```python
from build123d import *

# Parameters (mm, degrees)
SKETCH1_W           = 7
SKETCH1_H           = 2
SKETCH1_R           = 1
SKETCH1_W_2         = 23.5
SKETCH1_H_2         = 13
BOSS_EXTRUDE1_DEPTH = 2


with BuildPart() as part:
    # Sketch1 → Boss-Extrude1 (new body)
    with BuildSketch(Plane(origin=(0, 0, 0), x_dir=(1, 0, 0), z_dir=(0, 1, 0))):
        Polygon((66.949898611, 13.823848353), (-23.050101389, 13.823848353), (-23.050101389, 8.823848353), (-25.050101389, 8.823848353), (-25.050101389, 1.823848353), (-23.050101389, 1.823848353), (-23.050101389, -4.176151647), (-25.050101389, -4.176151647), (-25.050101389, -11.176151647), (-23.050101389, -11.176151647), (-23.050101389, -16.176151647), (66.949898611, -16.176151647), (66.949898611, -11.176151647), (68.949898611, -11.176151647), (68.949898611, -4.176151647), (66.949898611, -4.176151647), (66.949898611, 1.823848353), (68.949898611, 1.823848353), (68.949898611, 8.823848353), (66.949898611, 8.823848353), align=None)
        with Locations((-14.550101389, -7.676151647)):
            Rectangle(SKETCH1_W, SKETCH1_H, mode=Mode.SUBTRACT)
        with Locations(Location((1.699898611, -1.176151647, 0), (0, 0, 270))):
            Circle(SKETCH1_R, mode=Mode.SUBTRACT)
        with Locations((15.449898611, -1.176151647)):
            Rectangle(SKETCH1_W_2, SKETCH1_H_2, mode=Mode.SUBTRACT)
        with Locations(Location((29.199898611, -1.176151647, 0), (0, 0, 270))):
            Circle(SKETCH1_R, mode=Mode.SUBTRACT)
        with Locations((46.449898611, -7.676151647)):
            Rectangle(SKETCH1_W, SKETCH1_H, mode=Mode.SUBTRACT)
        with Locations((58.449898611, -7.676151647)):
            Rectangle(SKETCH1_W, SKETCH1_H, mode=Mode.SUBTRACT)
        Polygon((55.839898611, -0.11430823), (50.890151142, -5.064055698), (49.47593758, -3.649842135), (54.425685048, 1.299905333), align=None, mode=Mode.SUBTRACT)
        with Locations((-14.550101389, 5.323848353)):
            Rectangle(SKETCH1_W, SKETCH1_H, mode=Mode.SUBTRACT)
        with Locations((46.449898611, 5.323848353)):
            Rectangle(SKETCH1_W, SKETCH1_H, mode=Mode.SUBTRACT)
        with Locations((58.449898611, 5.323848353)):
            Rectangle(SKETCH1_W, SKETCH1_H, mode=Mode.SUBTRACT)
    extrude(amount=BOSS_EXTRUDE1_DEPTH)


solid = part.part
```
Here's how the part is built. I have some questions about the finished solid (model axes, mm). A direction names the side the tool comes from. Coordinates: 2 decimals unless noted, no trailing zeros. Order: outer loops, then holes, each group sorted by start corner. A loop starts at its lowest first (then second) coordinate and runs counter-clockwise, first axis right, second up. Notation, with made-up numbers: (-14, 18.25) - (44, 18.25) arc R20 cw to (44, 34.25) - close; hole circle Ø10 at (64.5, 40). An arc over 180 degrees is marked (long way). One line per question, with ' | ' between items. Start each with the question number.
1. Please list where these lines run through material, in increasing order: line 1 along X through (y, z) = (0.85, 8.5); line 2 along Z through (x, y) = (46.5, 1.5); line 3 along X through (y, z) = (0.3, -4). Write a range as [from, to].
2. If we section it at B-B (x = 48.5): Write out the boundary of the cut face in (y, z).
3. If we section it at D-D (y = 1.5): Give the number of separate pieces and of enclosed holes in the cut face, and give its area (3 significant figures).
4. If we section it at C-C (z = -10.5): Write out the boundary of the cut face in (x, y).
5. If we section it at A-A (z = -3.25): Write out the boundary of the cut face in (x, y).
6. Which directions (+Z, -Z, +X, -X, +Y, -Y) give clear straight access to the entire face, cutting with the end or side of a thin tool? Please do faces 5 (the flat face through (66.95, 1, 1)), 6 (the flat face through (-24, 1, 11.176)), 7 (the flat face through (61.95, 1, -5)).
7. I'm going to push a flat-ended pin straight in: pin 1 Ø0.6 at (x, y) = (-23.5, 0.5) entering from -Z. Where does the tip first touch, or does it pass through?
8. If we mould it in two halves opening along X, with no side actions, what happens to faces 1 (the flat face through (68.95, 1, -5)), 2 (the flat face through (68, 1, 4.176)), 3 (the flat face through (46, 1, -4.324)), 4 (the flat face through (58, 1, 6.676))? For each: released by +X, released by -X, zero draft, split by the parting line, or undercut.
Model answer:
1) line 1: x = [-25.05, -18.05], [-11.05, 42.95], [49.95, 54.95], [61.95, 68.95] | line 2: z = [-13.82, -6.32], [-4.32, 6.68], [8.68, 16.18] | line 3: x = [-25.05, 3.7], [27.2, 68.95]
2) outline: (0, -13.82) - (2, -13.82) - (2, -6.32) - (0, -6.32) - close; (0, -4.32) - (2, -4.32) - (2, 6.68) - (0, 6.68) - close; (0, 8.68) - (2, 8.68) - (2, 16.18) - (0, 16.18) - close
3) separate pieces: 1 | enclosed holes: 10 | area: 2,350 mm²
4) outline: (-23.05, 0) - (66.95, 0) - (66.95, 2) - (-23.05, 2) - close
5) outline: (-25.05, 0) - (3.7, 0) - (3.7, 2) - (-25.05, 2) - close; (27.2, 0) - (68.95, 0) - (68.95, 2) - (27.2, 2) - close
6) face 5: +X, +Y, -Y | face 6: +Z, -X, +Y, -Y | face 7: +Y, -Y
7) pin 1: stops at z = -8.82
8) face 1: released by +X | face 2: zero draft | face 3: undercut | face 4: undercut
